Check sheet for the modelled part. Datum: model origin and axes. Units: mm. A direction names the side the tool comes from. Give positions to 0.01 mm unless a question says otherwise; leave off trailing zeros. Write each loop counter-clockwise with the first axis right and the second up, starting at its lowest first coordinate (ties: lowest second). Pieces come first, ordered by that corner, then holes. Notation, with made-up numbers: (45, 23.25) -> (65, 23.25) arc R29 cw to (65, 45.25) -> close; hole circle Ø6 at (41.25, 23). An arc over 180 degrees is marked (long way). Return JSON: item names as keys, results as strings.
Autodesk Inventor part; units mm, degrees
ref_plane "YZ Plane" through (0, 0, 0) normal (1, 0, 0) x (0, 1, 0)
ref_plane "XZ Plane" through (0, 0, 0) normal (0, 1, 0) x (-1, 0, 0)
ref_plane "XY Plane" through (0, 0, 0) normal (0, 0, 1) x (1, 0, 0)
sketch "Sketch1" plane through (0, 0, 0) normal (0, 0, 1) x (1, 0, 0)
  line L0 (52.1089, 41.9337) -> (16.0623, 32.275)
  line L1 (81.0151, 18.2189) -> (81.0151, 29.0119)
  line L2 (81.0151, 29.0119) -> (52.1089, 36.7573)
  line L3 (52.1089, 36.7573) -> (16.0623, 27.0986)
  line L4 (16.0623, 32.275) -> (16.0623, 27.0986)
  line L5 (71.0038, 9.1932) -> (89.0623, 14.032)
  line L6 (71.0038, 9.1932) -> (54.0038, 9.1932)
  line L7 (54.0092, 15.1932) -> (69.7233, 15.1932)
  arc A0 (54.0092, 15.1932) -> (54.0038, 9.1932) centre (54.0065, 12.1932) ccw
  line L8 (69.7233, 15.1932) -> (81.0151, 18.2189)
  line L9 (52.1089, 41.9337) -> (89.0623, 32.032)
  line L10 (97.0623, 35.532) -> (97.0623, 10.532)
  circle A1 centre (94.2623, 31.5608) radius 1.35
  circle A2 centre (94.2623, 14.5608) radius 1.35
  line L11 (89.0623, 32.032) -> (91.4623, 32.032)
  line L12 (91.4623, 32.032) -> (91.4623, 35.532)
  line L13 (91.4623, 35.532) -> (97.0623, 35.532)
  line L14 (89.0623, 14.032) -> (91.4623, 14.032)
  line L15 (91.4623, 14.032) -> (91.4623, 10.532)
  line L16 (91.4623, 10.532) -> (97.0623, 10.532)
  point P0 (0, 0)
  dimension "d0" = 5
  dimension "d1" = 6
  dimension "d2" = 5
  dimension "d3" = 75
  dimension "d4" = 150
  dimension "d5" = 18
  dimension "d6" = 15
  dimension "d28" = 25
  dimension "d30" = 5.6
  dimension "d31" = 5.6
extrude "Extrusion1" add sketch "Sketch1" along normal blind 30
fillet "Fillet1" radius 3 7 edges at (81.0151, 29.0119, 15) (81.0151, 18.2189, 15) (69.7233, 15.1932, 15) (52.1089, 36.7573, 15) (52.1089, 41.9337, 15) (16.0623, 32.275, 15) (71.0038, 9.1932, 15)
sketch "Sketch7" plane through (0, 0, 30) normal (0, 0, 1) x (1, 0, 0)
  line L0 (81.0151, 20.5208) -> (47.1738, 20.5208)
  line L1 (47.1738, 20.5208) -> (47.1738, 6.5941)
  line L2 (47.1738, 6.5941) -> (81.0151, 6.5941)
  line L3 (81.0151, 6.5941) -> (81.0151, 20.5208)
  point P0 (0, 0)
extrude "Extrusion6" cut sketch "Sketch7" against normal blind 25
sketch "Sketch6" plane through (91.4623, 35.532, 0) normal (0, 1, 0) x (1, 0, 0)
  line L0 (0, 0) -> (0, -30)
  line L1 (5.6, 0) -> (0, 0)
  line L2 (0, 0) -> (0, -4.5)
  line L3 (0, -4.5) -> (5.6, -4.5)
  line L4 (5.6, -4.5) -> (5.6, 0)
  line L5 (5.6, -30) -> (0, -30)
  line L6 (0, -30) -> (0, -25.5)
  line L7 (0, -25.5) -> (5.6, -25.5)
  line L8 (5.6, -25.5) -> (5.6, -30)
  point P0 (-91.4623, 0)
  dimension "d32" = 4.5
  dimension "d33" = 5.6
  dimension "d34" = 4.5
extrude "Extrusion5" cut sketch "Sketch6" against normal through all
fillet "Fillet2" radius 3 2 edges at (91.4623, 14.032, 15) (91.4623, 32.032, 15)
properties part number "Left Hand" material "Aluminum-6061"
(1) Cross-section at C-C on z = 17.5. Enter the section's corners in (x, y).
Reply:
{"outline": "(16.06, 27.1) -> (51.33, 36.55) arc R3 cw to (52.89, 36.55) -> (78.79, 29.61) arc R3 cw to (81.02, 26.71) -> (81.02, 11.88) -> (89.06, 14.03) arc R3 cw to (91.46, 11.09) -> (91.46, 10.53) -> (97.06, 10.53) -> (97.06, 35.53) -> (91.46, 35.53) -> (91.46, 34.97) arc R3 cw to (89.06, 32.03) -> (52.89, 41.73) arc R3 ccw to (51.33, 41.73) -> (18.29, 32.87) arc R3 ccw to (16.06, 29.97) -> close; hole circle Ø2.7 at (94.26, 14.56); hole circle Ø2.7 at (94.26, 31.56)"}
(2) Cross-section at D-D on z = 2.75. Enter the section's corners in (x, y), then the cut area to 3 significant figures.
Reply:
{"outline": "(16.06, 27.1) -> (51.33, 36.55) arc R3 cw to (52.89, 36.55) -> (78.79, 29.61) arc R3 cw to (81.02, 26.71) -> (81.02, 20.52) arc R3 cw to (78.79, 17.62) -> (70.1, 15.3) arc R3 cw to (69.33, 15.19) -> (54.01, 15.19) arc R3 ccw to (54, 9.19) -> (70.61, 9.19) arc R3 ccw to (71.39, 9.3) -> (89.06, 14.03) -> (91.46, 14.03) -> (91.46, 32.03) -> (89.06, 32.03) -> (52.89, 41.73) arc R3 ccw to (51.33, 41.73) -> (18.29, 32.87) arc R3 ccw to (16.06, 29.97) -> close", "area": "722 mm^2"}
(3) Cross-section at B-B on x = 58.5. Enter the section's corners in (y, z), then the cut area to 3 significant figures.
Reply:
{"outline": "(9.19, 0) -> (15.19, 0) -> (15.19, 5) -> (9.19, 5) -> close; (35.04, 0) -> (40.22, 0) -> (40.22, 30) -> (35.04, 30) -> close", "area": "185 mm^2"}
(4) Depth check by flat-ended pin: pin 1 Ø3 at (x, y) = (94.26, 14.56) entering from +Z; pin 2 Ø1.5 at (x, z) = (42.5, 8.5) entering from +Y; pin 3 Ø1.3 at (y, z) = (25, 28) entering from +X. Enter the tip coordinate at first touch or a pass-through.
Reply:
{"pin 1": "z = 25.5", "pin 2": "y = 39.56", "pin 3": "x = 91.46"}
(5) Thickness scan on L1, parallel to Y at x = 92, z = 12.75; L2, parallel to X at y = 20.5, z = 22.75; L3, parallel to Z at x = 93.5, y = 20. Record the ranges inside material, lowest first.
Reply:
{"L1": "10.53 to 35.53", "L2": "81.02 to 97.06", "L3": "4.5 to 25.5"}
(6) Release check for a two-part mould opening along Y. For faces 4 (the cylindrical face through (95.5, 32.1, 14.9)), 5 (the flat face through (95, 23, 25.5)), 6 (the flat face through (90, 32.032, 2)) record: pulls with the +Y half, pulls with the -Y half, needs draft (parallel to the pull), parting line crosses it, or undercut.
Reply:
{"face 4": "undercut", "face 5": "needs draft", "face 6": "pulls with the +Y half"}
(7) Set-up check for faces 1 (the cylindrical face through (90.77, 13.01, 14.85)), 2 (the cylindrical face through (80.4, 18.7, 2.5)), 3 (the flat face through (91.462, 23, 2)): record each of +Z, -Z, +X, -X, +Y, -Y from which the full face is reachable in a straight line by a thin tool's end or side.
Reply:
{"face 1": "+Z, -Z, -Y", "face 2": "+Z, -Z, -X", "face 3": "-Z, +X, +Y, -Y"}
(8) Cross-section at A-A on y = 23. Enter the section's corners in (x, z).
Reply:
{"outline": "(81.02, 0) -> (91.46, 0) -> (91.46, 4.5) -> (97.06, 4.5) -> (97.06, 25.5) -> (91.46, 25.5) -> (91.46, 30) -> (81.02, 30) -> close"}
